Source: three-view drawing plus pictorial views. Frame: mm from the lowest corner of the part. A direction names the side the tool comes from. Coordinates: 2 decimals unless noted, no trailing zeros. Write each loop counter-clockwise with the first axis right and the second up, starting at its lowest first coordinate (ties: lowest second). Pieces come first, ordered by that corner, then holes. Notation, with made-up numbers: (-29.75, 0.5) - (-2.75, 0.5) arc R28 cw to (-2.75, 33.5) - close; hole circle Ø1 at (-21, 13). An arc over 180 degrees is marked (long way). Put each result on its own line as item: value. Start each with the question number.
1. Cut plane B-B, the plane z = 6.5. Return loops of the section in (x, y).
2. Cut plane D-D, the plane z = 2.25. Return loops of the section in (x, y), and give its area (3 significant figures).
3. Access query for the marked faces 1 and 2. Directions: +Z, -Z, +X, -X, +Y, -Y. A direction counts if a zero-diameter tool reaches every point of the face in a straight line with its end or side. Return the directions, or none.
4. Cut plane C-C, the plane y = 73. Return loops of the section in (x, z), and give its area (3 significant figures).
5. Line query: line 1 (Z direction, x = 5, y = 0.75); line 2 (X direction, y = 0.5, z = 6.5); line 3 (Z direction, x = 15, y = 0.65). Output: solid intervals per line, ascending.
6. Cut plane A-A, the plane x = 15. Return loops of the section in (y, z), and give its area (4 significant figures).
7. Pin query (flat end, axial travel): pin 1 (6 mm diameter, centred on y = 64.5, z = 3.5, fed in from +X); pin 2 (6 mm diameter, centred on x = 11.5, y = 69.5, fed in from -Z); pin 3 (5 mm diameter, centred on x = 11, z = 8, fed in from +Y); pin 4 (3 mm diameter, centred on x = 4, y = 47.5, fed in from +Z). Return the tip coordinate at first contact, or that it passes through.
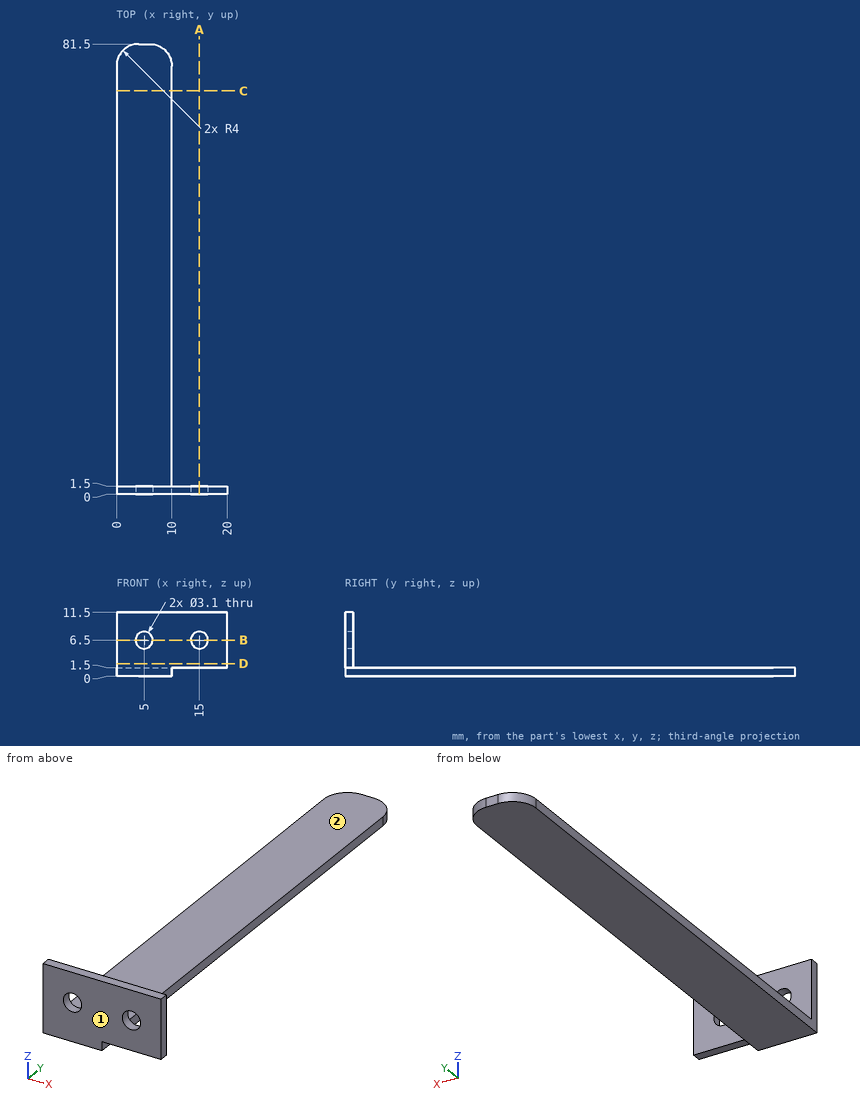
Report:
1. outline: (0, 0) - (3.45, 0) - (3.45, 1.5) - (0, 1.5) - close; (6.55, 0) - (13.45, 0) - (13.45, 1.5) - (6.55, 1.5) - close; (16.55, 0) - (20, 0) - (20, 1.5) - (16.55, 1.5) - close
2. outline: (0, 0) - (20, 0) - (20, 1.5) - (0, 1.5) - close
2. area: 30.0 mm^2
3. face 1: +Z, -Z, +X, -X, -Y
3. face 2: +Z, +X, -X, +Y
4. outline: (0, 0) - (10, 0) - (10, 1.5) - (0, 1.5) - close
4. area: 15.0 mm^2
5. line 1: z = 0 to 4.95, 8.05 to 11.5
5. line 2: x = 0 to 3.45, 6.55 to 13.45, 16.55 to 20
5. line 3: z = 1.5 to 4.95, 8.05 to 11.5
6. outline: (0, 1.5) - (1.5, 1.5) - (1.5, 4.95) - (0, 4.95) - close; (0, 8.05) - (1.5, 8.05) - (1.5, 11.5) - (0, 11.5) - close
6. area: 10.35 mm^2
7. pin 1: stops at x = 10
7. pin 2: stops at z = 0
7. pin 3: stops at y = 1.5
7. pin 4: stops at z = 1.5
